Geometry: see drawing. Coordinates: mm, zero at the bounding-box minimum. Give positions to 0.01 mm unless a question says otherwise; leave off trailing zeros. Use a Markdown table: item, result. Add a question column.
(1) Material intervals for L1, parallel to Y at x = 76, z = 10 (1 decimal); L2, parallel to X at y = 86.5, z = 1.75; L3, parallel to X at y = 83, z = 9 (1 decimal), sorted ascending.
(2) Pin query (flat end, axial travel): pin 1 Ø2 at (x, y) = (5.04, 5.74) entering from +Z. Return the tip coordinate at first contact, or that it passes through.
(3) Draft query along Z for the marked faces 1, 2 and 3. Return one class per face: released by +Z, released by -Z, zero draft, split by the parting line, or undercut.
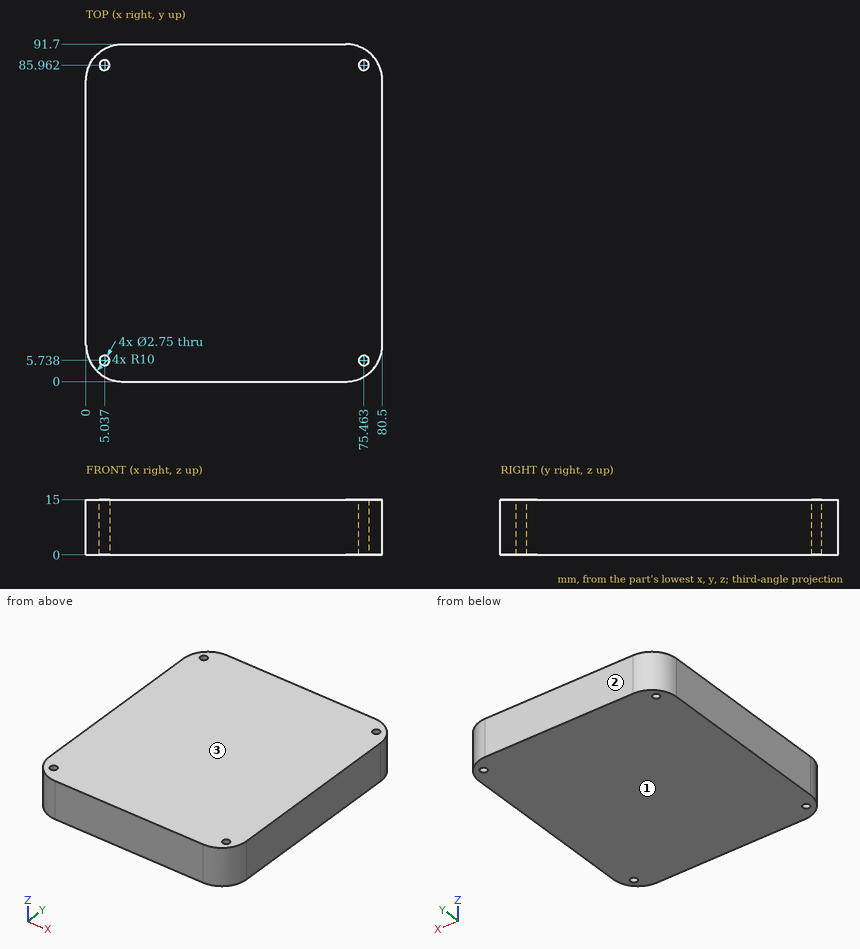
Answer list:
| question | item | result |
|---|---|---|
| 1 | L1 | 1.6 to 4.5, 7 to 84.7, 87.2 to 90.1 |
| 1 | L2 | 1.23 to 3.77, 6.3 to 74.2, 76.73 to 79.27 |
| 1 | L3 | 0.1 to 80.4 |
| 2 | pin 1 | through |
| 3 | face 1 | released by -Z |
| 3 | face 2 | zero draft |
| 3 | face 3 | released by +Z |
